Drawing for the job (mm, zero at the part's lowest x, y, z). Round coordinates to 2 decimals unless told otherwise and drop trailing zeros. Write each loop counter-clockwise with the first axis right and the second up, starting at its lowest first coordinate (ties: lowest second). Pieces come first, ordered by that corner, then holes. Notation, with made-up numbers: (-24, -25.5) - (-6, -25.5) arc R16 ccw to (-6, -10.5) - close; hole circle Ø5 at (-14.5, 70). An arc over 180 degrees is marked (long way). One line per question, with ' | ' between items.
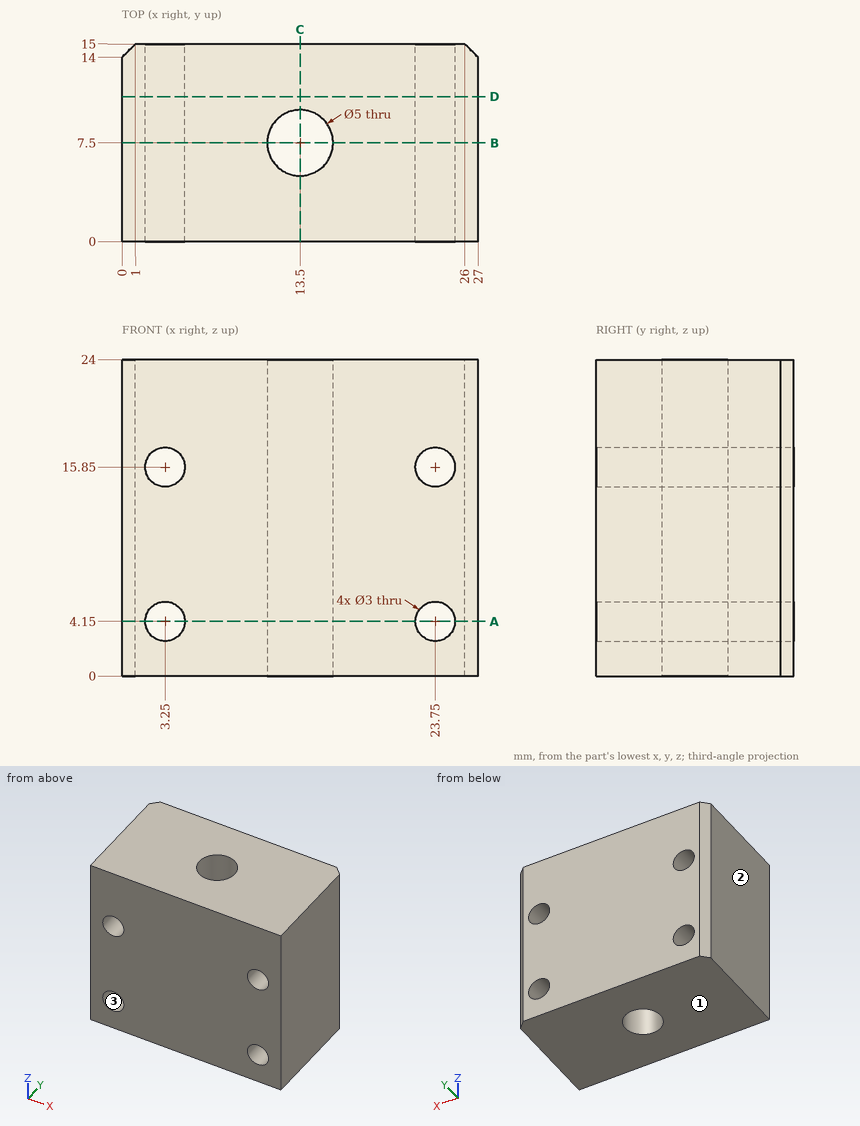
Q1. Saw through at D-D, the plane y = 11. List the corners of the cut face in (x, z), then the cut area to 3 significant figures.
Found:
outline: (0, 0) - (27, 0) - (27, 24) - (0, 24) - close; hole circle Ø3 at (3.25, 4.15); hole circle Ø3 at (3.25, 15.85); hole circle Ø3 at (23.75, 4.15); hole circle Ø3 at (23.75, 15.85) | area: 620 mm^2
Q2. Pull direction Z, two halves, no side cores. Call the marked faces 1, 2 and 3: +Z half, -Z half, draft (parallel to the pull), parting line (faces both ways), or undercut.
Found:
face 1: -Z half | face 2: draft | face 3: undercut
Q3. Saw through at B-B, the plane y = 7.5. List the corners of the cut face in (x, z), then the cut area to 3 significant figures.
Found:
outline: (0, 0) - (11, 0) - (11, 24) - (0, 24) - close; (16, 0) - (27, 0) - (27, 24) - (16, 24) - close; hole circle Ø3 at (3.25, 4.15); hole circle Ø3 at (3.25, 15.85); hole circle Ø3 at (23.75, 4.15); hole circle Ø3 at (23.75, 15.85) | area: 500 mm^2
Q4. Saw through at A-A, the plane z = 4.15. List the corners of the cut face in (x, y).
Found:
outline: (0, 0) - (1.75, 0) - (1.75, 15) - (1, 15) - (0, 14) - close; (4.75, 0) - (22.25, 0) - (22.25, 15) - (4.75, 15) - close; (25.25, 0) - (27, 0) - (27, 14) - (26, 15) - (25.25, 15) - close; hole circle Ø5 at (13.5, 7.5)
Q5. Drill centre lines: L1, parallel to Z at x = 23.75, y = 3; L2, parallel to X at y = 11.25, z = 15.85; L3, parallel to X at y = 6.25, z = 15.85. Where is each one in solid material? Low to high. Write a range as from..to.
Found:
L1: 0..2.65, 5.65..14.35, 17.35..24 | L2: 0..1.75, 4.75..22.25, 25.25..27 | L3: 0..1.75, 4.75..11.33, 15.67..22.25, 25.25..27
Q6. Saw through at C-C, the plane x = 13.5. List the corners of the cut face in (y, z).
Found:
outline: (0, 0) - (5, 0) - (5, 24) - (0, 24) - close; (10, 0) - (15, 0) - (15, 24) - (10, 24) - close
